Part model, mm, in its own coordinate system. A direction names the side the tool comes from. Coordinates: 2 decimals unless noted, no trailing zeros. Write each loop counter-clockwise with the first axis right and the second up, starting at its lowest first coordinate (ties: lowest second). Pieces come first, ordered by that corner, then holes. Notation, with made-up numbers: (11, 56.5) -> (67, 56.5) arc R23 ccw to (67, 69.5) -> close; hole circle Ø9 at (11, 49). An arc over 180 degrees is marked (long way). Write item = value, one per line.
from build123d import *

# Parameters (mm, degrees)
F0_W      = 30
F0_H      = 81
F1_DEPTH  = 2.1
F2_W      = 30
F2_H      = 2.1
F3_DEPTH  = 51.2
F4_W      = 30
F4_H      = 2.1
F5_DEPTH  = 13.1
F6_W      = 30
F6_H      = 2.1
F7_DEPTH  = 16
F8_W      = 10.1
F8_H      = 10.2
F9_DEPTH  = 2.1
F11_DEPTH = 15.201
F13_DEPTH = 2.101
F14_R     = 2.1
F14_R_2   = 1.6
F15_DEPTH = 2.101
F16_W     = 2.1
F16_H     = 12.85
F17_DEPTH = 30
F18_R     = 1.1
F19_DEPTH = 25


with BuildPart() as f1:
    # F0 (on Front) → F1 (new body)
    with BuildSketch(Plane.XZ):
        Rectangle(F0_W, F0_H)
    extrude(amount=F1_DEPTH)

    # F2 (on face) → F3 (join)
    with BuildSketch(Plane.XZ.offset(2.1)):
        with Locations((0, -39.45)):
            Rectangle(F2_W, F2_H)
    extrude(amount=F3_DEPTH)

    # F4 (on face) → F5 (join)
    with BuildSketch(Plane.XY.offset(-38.4)):
        with Locations((0, -52.25)):
            Rectangle(F4_W, F4_H)
    extrude(amount=F5_DEPTH)

    # F6 (on face) → F7 (join)
    with BuildSketch(Plane.XZ.offset(53.3)):
        with Locations((0, -26.35)):
            Rectangle(F6_W, F6_H)
    extrude(amount=F7_DEPTH)

    # F8 (on face) → F9 (join)
    with BuildSketch(Plane.XY.offset(-25.3)):
        with Locations((-20.05, -64.2)):
            Rectangle(F8_W, F8_H)
        with Locations((20.05, -64.2)):
            Rectangle(F8_W, F8_H)
    extrude(amount=-F9_DEPTH)

    # F10 (on face) → F11 (cut, through all)
    with BuildSketch(Plane.XY.offset(-25.3)):
        with BuildLine():
            Line((-21.9, -63.2), (-21.9, -65.2))
            ThreePointArc((-21.9, -65.2), (-20.3, -66.8), (-18.7, -65.2))
            Line((-18.7, -65.2), (-18.7, -63.2))
            ThreePointArc((-18.7, -63.2), (-20.3, -61.6), (-21.9, -63.2))
        make_face()
        with BuildLine():
            Line((18.7, -63.2), (18.7, -65.2))
            ThreePointArc((18.7, -65.2), (20.3, -66.8), (21.9, -65.2))
            Line((21.9, -65.2), (21.9, -63.2))
            ThreePointArc((21.9, -63.2), (20.3, -61.6), (18.7, -63.2))
        make_face()
    extrude(amount=-F11_DEPTH, mode=Mode.SUBTRACT)

    # F12 (on face) → F13 (cut, through all)
    with BuildSketch(Plane.XY.offset(-38.4)):
        with BuildLine():
            Line((-15, -22.894339), (-9.15, -22.894339))
            ThreePointArc((-9.15, -22.894339), (-4.15, -17.894339), (-9.15, -12.894339))
            Line((-9.15, -12.894339), (-15, -12.894339))
            Line((-15, -12.894339), (-15, -22.894339))
        make_face()
    extrude(amount=-F13_DEPTH, mode=Mode.SUBTRACT)

    # F14 (on face) → F15 (cut, through all)
    with BuildSketch(Plane.XZ.offset(2.1)):
        with Locations((9, 35.6)):
            Circle(F14_R)
        with Locations((9, 11.6)):
            Circle(F14_R)
        with Locations((-9, 35.6)):
            Circle(F14_R)
        with Locations((-9, 11.6)):
            Circle(F14_R)
        with Locations((9, -9.2)):
            Circle(F14_R)
        with Locations((-9, -9.2)):
            Circle(F14_R)
        with Locations((6.05, -0.7)):
            Circle(F14_R_2)
        with Locations((-6.05, -0.7)):
            Circle(F14_R_2)
    extrude(amount=-F15_DEPTH, mode=Mode.SUBTRACT)

    # F16 (on face) → F17 (join)
    with BuildSketch(Plane(origin=(-15, 0, 0), x_dir=(0, -1, 0), z_dir=(-1, 0, 0))):
        with Locations((1.05, 34.075)):
            Rectangle(F16_W, F16_H)
    extrude(amount=F17_DEPTH)

    # F18 (on face) → F19 (cut)
    with BuildSketch(Plane.XZ.offset(2.1)):
        with Locations((-42, 38.175)):
            Circle(F18_R)
        with Locations((-42, 29.975)):
            Circle(F18_R)
    extrude(amount=-F19_DEPTH, mode=Mode.SUBTRACT)


solid = f1.part
Q1. Probe line 1 (Z direction, x = 9, y = -1.25); line 2 (Y direction, x = -4.5, z = -29.5); line 3 (X direction, y = -1, z = 11). List the from-to ranges inside material, lowest first. Write a range as from..to.
Model answer:
line_1 = -40.5..-11.3, -7.1..9.5, 13.7..33.5, 37.7..40.5
line_2 = -53.3..-51.2, -2.1..0
line_3 = -15..-11.01, -6.99..6.99, 11.01..15
Q2. Saw through at A-A on z = 35.6. Give the cut face in (x, y).
Model answer:
outline = (-45, -2.1) -> (-11.1, -2.1) -> (-11.1, 0) -> (-45, 0) -> close; (-6.9, -2.1) -> (6.9, -2.1) -> (6.9, 0) -> (-6.9, 0) -> close; (11.1, -2.1) -> (15, -2.1) -> (15, 0) -> (11.1, 0) -> close
Q3. Saw through at D-D on x = 20.3. Give the cut face in (y, z), and give its area (3 significant figures).
Model answer:
outline = (-69.3, -27.4) -> (-66.8, -27.4) -> (-66.8, -25.3) -> (-69.3, -25.3) -> close; (-61.6, -27.4) -> (-59.1, -27.4) -> (-59.1, -25.3) -> (-61.6, -25.3) -> close
area = 10.5 mm²
Q4. Which spindle directions (+Z, -Z, +X, -X, +Y, -Y) get a long thin tool onto all of the face, cutting with end or side? Do faces 4 (the face through (-1, -2.1, 0)), 5 (the face through (-12, -12.894, -39)), 6 (the face through (0, -53.3, -34)), 7 (the face through (-20, -59.1, -26)), 8 (the face through (-30, -1, 27.65)). Say none if no direction does.
Model answer:
face_4 = +Z, +X, -X
face_5 = +Z, -Z, -X
face_6 = -Z, +X, -X, -Y
face_7 = +Z, -Z, -X, +Y
face_8 = -Z, -X, +Y, -Y
Q5. Pin check, flat tips, straight feed: pin 1 (2 mm diameter, centred on y = -64.5, z = -26, fed in from -X); pin 2 (0.6 mm diameter, centred on x = 19, z = -26, fed in from +Y); pin 3 (8 mm diameter, centred on x = 8.5, y = -28.5, fed in from +Z); pin 4 (5 mm diameter, centred on x = -25.5, z = -31.5, fed in from +Y). Stop position of each tip, or through.
Model answer:
pin_1 = -25.1
pin_2 = -59.1
pin_3 = -38.4
pin_4 = through
Q6. Saw through at B-B on x = -42. Give the cut face in (y, z) (3 decimals), and give its area (3 significant figures).
Model answer:
outline = (-2.1, 27.65) -> (0, 27.65) -> (0, 28.875) -> (-2.1, 28.875) -> close; (-2.1, 31.075) -> (0, 31.075) -> (0, 37.075) -> (-2.1, 37.075) -> close; (-2.1, 39.275) -> (0, 39.275) -> (0, 40.5) -> (-2.1, 40.5) -> close
area = 17.7 mm²
Q7. Mould opens along X. For faces 1 (the face through (7.452, -1.065, 13.019)), 2 (the face through (-1, 0, -1)), 3 (the face through (-45, -1, 34)) say: released by +X, released by -X, zero draft, split by the parting line, or undercut.
Model answer:
face_1 = undercut
face_2 = zero draft
face_3 = released by -X
Q8. Saw through at C-C on z = -29. Give the cut face in (x, y), and give its area (3 significant figures).
Model answer:
outline = (-15, -53.3) -> (15, -53.3) -> (15, -51.2) -> (-15, -51.2) -> close; (-15, -2.1) -> (15, -2.1) -> (15, 0) -> (-15, 0) -> close
area = 126 mm²
